```python
from build123d import *

# Parameters (mm, degrees)
SKETCH1_W           = 190
SKETCH1_H           = 385
SKETCH1_R           = 5
SKETCH1_R_2         = 1.5
BOSS_EXTRUDE1_DEPTH = 2


with BuildPart() as part:
    # Sketch1 → Boss-Extrude1 (new body)
    with BuildSketch(Plane(origin=(0, 0, 0), x_dir=(1, 0, 0), z_dir=(0, 1, 0))):
        Rectangle(SKETCH1_W, SKETCH1_H)
        with Locations(Location((-59.69, -168.55, 0), (0, 0, 270))):
            Circle(SKETCH1_R, mode=Mode.SUBTRACT)
        with Locations(Location((-44.45, -168.55, 0), (0, 0, 270))):
            Circle(SKETCH1_R, mode=Mode.SUBTRACT)
        with Locations(Location((-29.21, -168.55, 0), (0, 0, 270))):
            Circle(SKETCH1_R, mode=Mode.SUBTRACT)
        with Locations(Location((-13.97, -168.55, 0), (0, 0, 270))):
            Circle(SKETCH1_R, mode=Mode.SUBTRACT)
        with Locations(Location((1.27, -168.55, 0), (0, 0, 270))):
            Circle(SKETCH1_R, mode=Mode.SUBTRACT)
        with Locations(Location((16.51, -168.55, 0), (0, 0, 270))):
            Circle(SKETCH1_R, mode=Mode.SUBTRACT)
        with Locations(Location((31.75, -168.55, 0), (0, 0, 270))):
            Circle(SKETCH1_R, mode=Mode.SUBTRACT)
        with Locations(Location((46.99, -168.55, 0), (0, 0, 270))):
            Circle(SKETCH1_R, mode=Mode.SUBTRACT)
        with Locations(Location((64.77, -168.55, 0), (0, 0, 270))):
            Circle(SKETCH1_R, mode=Mode.SUBTRACT)
        with Locations(Location((64.77, -148.27, 0), (0, 0, 270))):
            Circle(SKETCH1_R, mode=Mode.SUBTRACT)
        with Locations(Location((-71.93, 178.11, 0), (0, 0, 270))):
            Circle(SKETCH1_R_2, mode=Mode.SUBTRACT)
        with Locations(Location((71.93, 178.11, 0), (0, 0, 270))):
            Circle(SKETCH1_R_2, mode=Mode.SUBTRACT)
        with Locations(Location((71.93, -178.11, 0), (0, 0, 270))):
            Circle(SKETCH1_R_2, mode=Mode.SUBTRACT)
        with Locations(Location((-71.93, -178.11, 0), (0, 0, 270))):
            Circle(SKETCH1_R_2, mode=Mode.SUBTRACT)
    extrude(amount=BOSS_EXTRUDE1_DEPTH)


solid = part.part
```
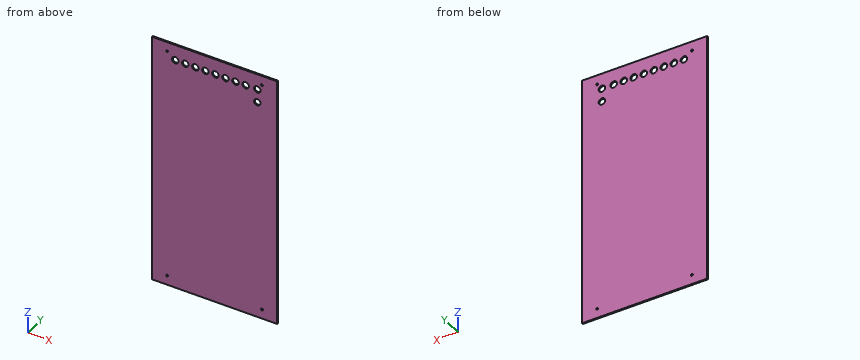
Verification items for the finished model (mm, model axes). Round coordinates to 2 decimals unless told otherwise and drop trailing zeros. Write each loop counter-clockwise with the first axis right and the second up, starting at its lowest first coordinate (ties: lowest second). Pieces come first, ordered by that corner, then holes.
1. Scan lines: L1, parallel to X at y = 0.65, z = 178.11; L2, parallel to Z at x = 71.93, y = 1.45; L3, parallel to Z at x = 61, y = 1.1. Record each from-to range of solid material in increasing order.
2. Section check B-B on z = 168.55. State how many separate pieces and enclosed holes the cut face has, plus the area to 3 significant figures.
3. Gauge pin test, flat end, axial feed: P1, Ø6, axis at x = -29.21, z = 168.55, coming from the -Y side. Record the tip position at first contact, or that the pin passes through.
4. Section check A-A on x = 1.27. Enter the section's corners in (y, z), plus the area to 3 significant figures.
Answer:
1. L1: x = -95 to -73.43, -70.43 to 70.43, 73.43 to 95
1. L2: z = -192.5 to -179.61, -176.61 to 176.61, 179.61 to 192.5
1. L3: z = -192.5 to 144.99, 151.55 to 165.27, 171.83 to 192.5
2. separate pieces: 10
2. enclosed holes: 0
2. area: 200 mm2
3. P1: passes through
4. outline: (0, -192.5) - (2, -192.5) - (2, 163.55) - (0, 163.55) - close; (0, 173.55) - (2, 173.55) - (2, 192.5) - (0, 192.5) - close
4. area: 750 mm2
